```python
from build123d import *

# Parameters (mm, degrees)
F0_W     = 60
F0_H     = 180
F0_R     = 1.6
F0_R_2   = 1.5
F1_DEPTH = 0.815


with BuildPart() as f1:
    # F0 (on Front) → F1 (new body, symmetric)
    with BuildSketch(Plane.XZ):
        with Locations((0, 93)):
            Rectangle(F0_W, F0_H)
        with Locations((-20, 23)):
            Circle(F0_R, mode=Mode.SUBTRACT)
        with Locations((0, 23)):
            Circle(F0_R_2, mode=Mode.SUBTRACT)
        with Locations((20, 23)):
            Circle(F0_R, mode=Mode.SUBTRACT)
    extrude(amount=F1_DEPTH, both=True)


solid = f1.part
```
Part model, mm, in its own coordinate system. Give positions to 0.01 mm unless a question says otherwise; leave off trailing zeros. Order: outer loops, then holes, each group sorted by start corner. A loop starts at its lowest first (then second) coordinate and runs counter-clockwise, first axis right, second up. Notation, with made-up numbers: M 6.25,-38.5 L 49.25,-38.5 A28 cw 49.25,-3.5 Z; hole C 54,82.5 d10. An arc over 180 degrees is marked long. Use a Markdown table: item, result. Add a question column.
(1) Probe line 1 along Z through (x, y) = (-20, 0.4); line 2 along Z through (x, y) = (0, 0.25). List the from-to ranges inside material, lowest first. Write a range as [from, to].
(2) Drop a flat-ended pin along its axis: P1, Ø3.5, axis at x = 20, z = 23, coming from the -Y side (3 decimals). Give the stop position or say it passes through.
(3) Saw through at A-A, the plane x = 20. Give the cut face in (y, z) (3 decimals), and give its area (3 significant figures).
(4) Mould opens along Z. For faces 1 (the face through (-0.195, 0.011, 24.487)), 2 (the face through (0, 0.815, 94)) say: +Z half, -Z half, draft (parallel to the pull), parting line (faces both ways), or undercut.
Answer key:
| question | item | result |
|---|---|---|
| 1 | line 1 | [3, 21.4], [24.6, 183] |
| 1 | line 2 | [3, 21.5], [24.5, 183] |
| 2 | P1 | y = -0.815 |
| 3 | outline | M -0.815,3 L 0.815,3 L 0.815,21.4 L -0.815,21.4 Z; M -0.815,24.6 L 0.815,24.6 L 0.815,183 L -0.815,183 Z |
| 3 | area | 288 mm^2 |
| 4 | face 1 | undercut |
| 4 | face 2 | draft |
